from build123d import *
from OCP.BRepFilletAPI import BRepFilletAPI_MakeChamfer

# Parameters (mm, degrees)
BOSS_EXTRUDE1_DEPTH = 22
SKETCH2_R           = 7.95
BOSS_EXTRUDE2_DEPTH = 8
SKETCH3_OUTSIDE_W   = 32.288
SKETCH3_OUTSIDE_H   = 29.348
SKETCH3_OUTSIDE_R   = 9
CUT_EXTRUDE1_DEPTH  = 2
FILLET1_R           = 2
CHAMFER1_SIZE       = 2
FILLET2_R           = 2
CUT_EXTRUDE2_START  = -5
SKETCH4_OUTSIDE_W   = 31.604
SKETCH4_OUTSIDE_H   = 29.284
SKETCH4_OUTSIDE_R   = 8.5
CUT_EXTRUDE2_DEPTH  = 6
SKETCH5_R           = 4
CUT_EXTRUDE3_DEPTH  = 3
FILLET3_R           = 2
SKETCH6_R           = 5
CUT_EXTRUDE4_DEPTH  = 19
SKETCH7_R           = 0.7
CUT_EXTRUDE5_DEPTH  = 31.543264727
CHAMFER2_SIZE       = 0.5
CHAMFER2_SIZE2      = 0.288675135
SKETCH9_R           = 4
CUT_EXTRUDE6_DEPTH  = 31.543264727


with BuildPart() as part:
    # Sketch1 → Boss-Extrude1 (new body)
    with BuildSketch(Plane.XY):
        Polygon((10.969655115, 0), (5.484827557, 9.5), (-5.484827557, 9.5), (-10.969655115, 0), (-5.484827557, -9.5), (5.484827557, -9.5), align=None)
    extrude(amount=BOSS_EXTRUDE1_DEPTH)

    # Sketch2 → Boss-Extrude2 (add)
    with BuildSketch(Plane(origin=(0, 0, 0), x_dir=(-1, 0, 0), z_dir=(0, 0, -1))):
        Circle(SKETCH2_R)
    extrude(amount=BOSS_EXTRUDE2_DEPTH)

    # Sketch3 outside → Cut-Extrude1 (cut)
    with BuildSketch(Plane.XY.offset(22)):
        Rectangle(SKETCH3_OUTSIDE_W, SKETCH3_OUTSIDE_H)
        Circle(SKETCH3_OUTSIDE_R, mode=Mode.SUBTRACT)
    extrude(amount=-CUT_EXTRUDE1_DEPTH, mode=Mode.SUBTRACT)

    # Fillet1
    fillet1_edges = [part.edges().sort_by_distance(p)[0] for p in [
        (5.484827557, -9.5, 10),
        (-5.484827557, -9.5, 10),
        (-10.969655115, 0, 10),
        (-5.484827557, 9.5, 10),
        (5.484827557, 9.5, 10),
        (10.969655115, 0, 10),
    ]]
    fillet(fillet1_edges, radius=FILLET1_R)

    # Chamfer1
    # the kernel refuses this chamfer: 2 mm, written as the material it takes off along each edge
    with BuildSketch(Plane(origin=(-4.330127019, -9.5, 20), x_dir=(0, 1, 0), z_dir=(1, 0, 0))) as chamfer1_piece_1_section:
        Polygon((CHAMFER1_SIZE, 0), (0, -CHAMFER1_SIZE), (0, 0), align=None)
    chamfer1_piece_1 = extrude(amount=8.660254038, mode=Mode.PRIVATE)
    chamfer1_piece_1 = chamfer1_piece_1 - Plane(origin=(0, 0, 20), x_dir=(1, 0, 0), z_dir=(0, 0, 1)) * Cylinder(9, 26, mode=Mode.PRIVATE)
    add(chamfer1_piece_1, mode=Mode.SUBTRACT)
    with BuildSketch(Plane(origin=(4.330127019, -7.5, 20), x_dir=(0.8660254037844417, -0.49999999999999456, 0), z_dir=(0.49999999999999456, 0.8660254037844417, 0))) as chamfer1_piece_2_section:
        Polygon((2 - CHAMFER1_SIZE, 0), (2, CHAMFER1_SIZE), (2, 0), align=None)
    chamfer1_piece_2 = revolve(axis=Axis((4.330127019, -7.5, 20), (0, 0, -1)), revolution_arc=60, mode=Mode.PRIVATE)
    chamfer1_piece_2 = chamfer1_piece_2 - Plane(origin=(0, 0, 20), x_dir=(1, 0, 0), z_dir=(0, 0, 1)) * Cylinder(9, 8, mode=Mode.PRIVATE)
    add(chamfer1_piece_2, mode=Mode.SUBTRACT)
    with BuildSketch(Plane(origin=(-4.330127019, -7.5, 20), x_dir=(0, -1, 0), z_dir=(1, 0, 0))) as chamfer1_piece_3_section:
        Polygon((2 - CHAMFER1_SIZE, 0), (2, CHAMFER1_SIZE), (2, 0), align=None)
    chamfer1_piece_3 = revolve(axis=Axis((-4.330127019, -7.5, 20), (0, 0, -1)), revolution_arc=60, mode=Mode.PRIVATE)
    chamfer1_piece_3 = chamfer1_piece_3 - Plane(origin=(0, 0, 20), x_dir=(1, 0, 0), z_dir=(0, 0, 1)) * Cylinder(9, 8, mode=Mode.PRIVATE)
    add(chamfer1_piece_3, mode=Mode.SUBTRACT)
    with BuildSketch(Plane(origin=(6.062177826, -8.5, 20), x_dir=(-0.8660254037844416, 0.499999999999995, 0), z_dir=(0.499999999999995, 0.8660254037844416, 0))) as chamfer1_piece_4_section:
        Polygon((CHAMFER1_SIZE, 0), (0, -CHAMFER1_SIZE), (0, 0), align=None)
    chamfer1_piece_4 = extrude(amount=8.660254038, mode=Mode.PRIVATE)
    chamfer1_piece_4 = chamfer1_piece_4 - Plane(origin=(0, 0, 20), x_dir=(1, 0, 0), z_dir=(0, 0, 1)) * Cylinder(9, 26, mode=Mode.PRIVATE)
    add(chamfer1_piece_4, mode=Mode.SUBTRACT)
    with BuildSketch(Plane(origin=(-10.392304845, -1, 20), x_dir=(0.8660254037844345, 0.5000000000000072, 0), z_dir=(0.5000000000000072, -0.8660254037844346, 0))) as chamfer1_piece_5_section:
        Polygon((CHAMFER1_SIZE, 0), (0, -CHAMFER1_SIZE), (0, 0), align=None)
    chamfer1_piece_5 = extrude(amount=8.660254038, mode=Mode.PRIVATE)
    chamfer1_piece_5 = chamfer1_piece_5 - Plane(origin=(0, 0, 20), x_dir=(1, 0, 0), z_dir=(0, 0, 1)) * Cylinder(9, 26, mode=Mode.PRIVATE)
    add(chamfer1_piece_5, mode=Mode.SUBTRACT)
    with BuildSketch(Plane(origin=(8.660254038, 0, 20), x_dir=(0.866025403784438, 0.500000000000001, 0), z_dir=(-0.500000000000001, 0.866025403784438, 0))) as chamfer1_piece_6_section:
        Polygon((2, CHAMFER1_SIZE), (2 - CHAMFER1_SIZE, 0), (2, 0), align=None)
    chamfer1_piece_6 = revolve(axis=Axis((8.660254038, 0, 20), (0, 0, -1)), revolution_arc=60, mode=Mode.PRIVATE)
    chamfer1_piece_6 = chamfer1_piece_6 - Plane(origin=(0, 0, 20), x_dir=(1, 0, 0), z_dir=(0, 0, 1)) * Cylinder(9, 9, mode=Mode.PRIVATE)
    add(chamfer1_piece_6, mode=Mode.SUBTRACT)
    with BuildSketch(Plane(origin=(-8.660254038, 0, 20), x_dir=(-0.8660254037844414, 0.4999999999999952, 0), z_dir=(0.4999999999999952, 0.8660254037844414, 0))) as chamfer1_piece_7_section:
        Polygon((2 - CHAMFER1_SIZE, 0), (2, -CHAMFER1_SIZE), (2, 0), align=None)
    chamfer1_piece_7 = revolve(axis=Axis((-8.660254038, 0, 20), (0, 0, 1)), revolution_arc=60, mode=Mode.PRIVATE)
    chamfer1_piece_7 = chamfer1_piece_7 - Plane(origin=(0, 0, 20), x_dir=(1, 0, 0), z_dir=(0, 0, 1)) * Cylinder(9, 8, mode=Mode.PRIVATE)
    add(chamfer1_piece_7, mode=Mode.SUBTRACT)
    with BuildSketch(Plane(origin=(10.392304845, 1, 20), x_dir=(0, 0, -1), z_dir=(-0.500000000000001, 0.866025403784438, 0))) as chamfer1_piece_8_section:
        Polygon((CHAMFER1_SIZE, 0), (0, CHAMFER1_SIZE), (0, 0), align=None)
    chamfer1_piece_8 = extrude(amount=8.660254038, mode=Mode.PRIVATE)
    chamfer1_piece_8 = chamfer1_piece_8 - Plane(origin=(0, 0, 20), x_dir=(1, 0, 0), z_dir=(0, 0, 1)) * Cylinder(9, 26, mode=Mode.PRIVATE)
    add(chamfer1_piece_8, mode=Mode.SUBTRACT)
    with BuildSketch(Plane(origin=(-6.062177826, 8.5, 20), x_dir=(0.8660254037844415, -0.49999999999999517, 0), z_dir=(-0.49999999999999517, -0.8660254037844415, 0))) as chamfer1_piece_9_section:
        Polygon((CHAMFER1_SIZE, 0), (0, -CHAMFER1_SIZE), (0, 0), align=None)
    chamfer1_piece_9 = extrude(amount=8.660254038, mode=Mode.PRIVATE)
    chamfer1_piece_9 = chamfer1_piece_9 - Plane(origin=(0, 0, 20), x_dir=(1, 0, 0), z_dir=(0, 0, 1)) * Cylinder(9, 26, mode=Mode.PRIVATE)
    add(chamfer1_piece_9, mode=Mode.SUBTRACT)
    with BuildSketch(Plane(origin=(4.330127019, 7.5, 20), x_dir=(0.8660254037844379, 0.5000000000000013, 0), z_dir=(0.5000000000000013, -0.8660254037844379, 0))) as chamfer1_piece_10_section:
        Polygon((2, -CHAMFER1_SIZE), (2 - CHAMFER1_SIZE, 0), (2, 0), align=None)
    chamfer1_piece_10 = revolve(axis=Axis((4.330127019, 7.5, 20), (0, 0, 1)), revolution_arc=60, mode=Mode.PRIVATE)
    chamfer1_piece_10 = chamfer1_piece_10 - Plane(origin=(0, 0, 20), x_dir=(1, 0, 0), z_dir=(0, 0, 1)) * Cylinder(9, 9, mode=Mode.PRIVATE)
    add(chamfer1_piece_10, mode=Mode.SUBTRACT)
    with BuildSketch(Plane(origin=(-4.330127019, 7.5, 20), x_dir=(0, 1, 0), z_dir=(1, 0, 0))) as chamfer1_piece_11_section:
        Polygon((2 - CHAMFER1_SIZE, 0), (2, -CHAMFER1_SIZE), (2, 0), align=None)
    chamfer1_piece_11 = revolve(axis=Axis((-4.330127019, 7.5, 20), (0, 0, 1)), revolution_arc=60, mode=Mode.PRIVATE)
    chamfer1_piece_11 = chamfer1_piece_11 - Plane(origin=(0, 0, 20), x_dir=(1, 0, 0), z_dir=(0, 0, 1)) * Cylinder(9, 8, mode=Mode.PRIVATE)
    add(chamfer1_piece_11, mode=Mode.SUBTRACT)
    with BuildSketch(Plane(origin=(4.330127019, 9.5, 20), x_dir=(0, -1, 0), z_dir=(-1, 0, 0))) as chamfer1_piece_12_section:
        Polygon((CHAMFER1_SIZE, 0), (0, -CHAMFER1_SIZE), (0, 0), align=None)
    chamfer1_piece_12 = extrude(amount=8.660254038, mode=Mode.PRIVATE)
    chamfer1_piece_12 = chamfer1_piece_12 - Plane(origin=(0, 0, 20), x_dir=(1, 0, 0), z_dir=(0, 0, 1)) * Cylinder(9, 26, mode=Mode.PRIVATE)
    add(chamfer1_piece_12, mode=Mode.SUBTRACT)

    # Fillet2
    # the kernel refuses this fillet: 2 mm, written as the material it takes off along each edge
    with BuildSketch(Plane(origin=(0, 0, 22), x_dir=(1, 0, 0), z_dir=(0, -1, 0))) as fillet2_piece_1:
        with BuildLine():
            CenterArc((9 - FILLET2_R, -FILLET2_R), FILLET2_R, 0, 90)
            Line((9 - FILLET2_R, 0), (9, 0))
            Line((9, 0), (9, -FILLET2_R))
        make_face()
    revolve(axis=Axis((0, 0, 22), (0, 0, 1)), mode=Mode.SUBTRACT)

    # Sketch4 outside → Cut-Extrude2 (cut)
    with BuildSketch(Plane(origin=(0, 0, 0), x_dir=(-1, 0, 0), z_dir=(0, 0, -1)).offset(CUT_EXTRUDE2_START)):
        Rectangle(SKETCH4_OUTSIDE_W, SKETCH4_OUTSIDE_H)
        Circle(SKETCH4_OUTSIDE_R, mode=Mode.SUBTRACT)
    extrude(amount=-CUT_EXTRUDE2_DEPTH, mode=Mode.SUBTRACT)

    # Sketch5 → Cut-Extrude3 (cut)
    with BuildSketch(Plane.XY.offset(22)):
        Circle(SKETCH5_R)
    extrude(amount=-CUT_EXTRUDE3_DEPTH, mode=Mode.SUBTRACT)

    # Fillet3
    fillet3_edges = [part.edges().sort_by_distance(p)[0] for p in [
        (-4, 0, 22),
    ]]
    fillet(fillet3_edges, radius=FILLET3_R)

    # Sketch6 → Cut-Extrude4 (cut)
    with BuildSketch(Plane(origin=(0, 0, -8), x_dir=(-1, 0, 0), z_dir=(0, 0, -1))):
        Circle(SKETCH6_R)
    extrude(amount=-CUT_EXTRUDE4_DEPTH, mode=Mode.SUBTRACT)

    # Sketch7 → Cut-Extrude5 (cut, through all)
    with BuildSketch(Plane.XY.offset(19)):
        with Locations((-2.5, 0)):
            Circle(SKETCH7_R)
        with Locations((-1.25, 2.165063509)):
            Circle(SKETCH7_R)
        with Locations((1.25, 2.165063509)):
            Circle(SKETCH7_R)
        with Locations((2.5, 0)):
            Circle(SKETCH7_R)
        with Locations((1.25, -2.165063509)):
            Circle(SKETCH7_R)
        with Locations((-1.25, -2.165063509)):
            Circle(SKETCH7_R)
    extrude(amount=-CUT_EXTRUDE5_DEPTH, mode=Mode.SUBTRACT)

    # Sketch8 → Cut-Revolve1 (revolve, cut)
    with BuildSketch(Plane(origin=(0, 0, 0), x_dir=(1, 0, 0), z_dir=(0, 1, 0)), mode=Mode.PRIVATE) as cut_revolve1_sk:
        with BuildLine():
            Line((-6.75, 0.875), (-7.95, 0.875))
            Line((-7.95, 0.875), (-7.95, -0.625))
            Line((-7.95, -0.625), (-6.75, -0.625))
            ThreePointArc((-6.75, -0.625), (-6, 0.125), (-6.75, 0.875))
        make_face()
    revolve(cut_revolve1_sk.sketch.rotate(Axis((0, 0, 0), (0, 0, -1)), 180), axis=Axis((0, 0, 0), (0, 0, -1)), mode=Mode.SUBTRACT)

    # Chamfer2: one chamfer whose edges measure the first distance from different faces: ONE call of the kernel's chamfer builder (chamfer() names one face for all edges)
    chamfer2_edges_1 = [part.edges().sort_by_distance(p)[0] for p in [
        (-7.95, 0, 0),
    ]]
    chamfer2_side_1 = [part.faces().sort_by_distance(p)[0] for p in [
        (7.979921088, 4.607209589, 0),
    ]]
    chamfer2_edges_2 = [part.edges().sort_by_distance(p)[0] for p in [
        (7.95, 0, -0.875),
    ]]
    chamfer2_side_2 = [part.faces().sort_by_distance(p)[0] for p in [
        (7.95, 0, -4.4375),
    ]]
    chamfer2 = BRepFilletAPI_MakeChamfer(part.part.solid().wrapped)
    for e in chamfer2_edges_1:
        chamfer2.Add(CHAMFER2_SIZE, CHAMFER2_SIZE2, e.wrapped, chamfer2_side_1[0].wrapped)  # the first distance lies on this face
    for e in chamfer2_edges_2:
        chamfer2.Add(CHAMFER2_SIZE, CHAMFER2_SIZE2, e.wrapped, chamfer2_side_2[0].wrapped)  # the first distance lies on this face
    add(Compound.cast(chamfer2.Shape()), mode=Mode.REPLACE)

    # Sketch9 → Cut-Extrude6 (cut, through all)
    with BuildSketch(Plane.XY.offset(19)):
        Circle(SKETCH9_R)
    extrude(amount=-CUT_EXTRUDE6_DEPTH, mode=Mode.SUBTRACT)


solid = part.part
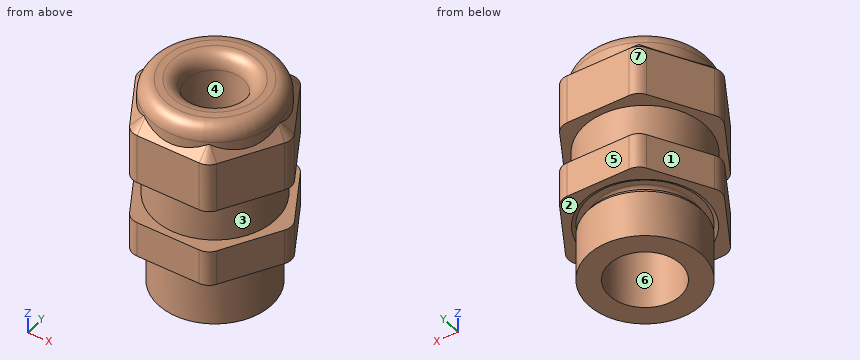
Here's how the part is built. I have some questions about the finished solid (model axes, mm). Face numbers are marked on the shaded views. A direction names the side the tool comes from. Coordinates: 2 decimals unless noted, no trailing zeros. Write each loop counter-clockwise with the first axis right and the second up, starting at its lowest first coordinate (ties: lowest second). Pieces come first, ordered by that corner, then holes. Notation, with made-up numbers: (7, 19) - (63, 19) arc R32 cw to (63, 58) - close; hole circle Ø10 at (24, -26.75). An arc over 180 degrees is marked (long way). Use one line per item in the form item = value.
1) I'm going to push flat-ended pins straight in: P1, Ø10.5, axis at x = 0, y = 0, coming from the +Z side; P2, Ø10, axis at y = 6.5, z = 15, coming from the +X side; P3, Ø2, axis at y = -2, z = 5, coming from the +X side. Where does each tip first touch, or does it pass through?
Solved:
P1 = 21.85
P2 = 10.1
P3 = 10.39
2) I need wall thicknesses on line 1 (Y direction, x = 0, z = 0.4); line 2 (Y direction, x = 0, z = 17.5); line 3 (Y direction, x = 0, z = 6.25). Which ranges of each line are inside material? Lowest first, please.
Solved:
line_1 = -9.5 to -7.95, -6.21 to -5, 5 to 6.21, 7.95 to 9.5
line_2 = -9.5 to -4, 4 to 9.5
line_3 = -8.5 to -5, 5 to 8.5
3) Suppose I cut it at A-A, the plane z = 2. Write out the boundary of the cut face in (x, y), plus the area to 3 significant figures.
Solved:
outline = (-10.39, -1) - (-6.06, -8.5) arc R2 ccw to (-4.33, -9.5) - (4.33, -9.5) arc R2 ccw to (6.06, -8.5) - (10.39, -1) arc R2 ccw to (10.39, 1) - (6.06, 8.5) arc R2 ccw to (4.33, 9.5) - (-4.33, 9.5) arc R2 ccw to (-6.06, 8.5) - (-10.39, 1) arc R2 ccw to start; hole circle Ø10 at (0, 0)
area = 233 mm2
4) Thinking about a two-plate mould opening in X: for the marked faces 4, 5, 6 and 7, which applies, released by +X, released by -X, zero draft, split by the parting line, or undercut?
Solved:
face_4 = undercut
face_5 = zero draft
face_6 = undercut
face_7 = released by -X
5) On a 3-axis mill with a long thin cutter (end or side, diameter ignored), from which of +Z, -Z, +X, -X, +Y, -Y can I reach the whole of each face in a straight line? I mean the marked faces 1, 2 and 3. Say none if no direction works.
Solved:
face_1 = +Z, -Z, -X, +Y
face_2 = -Z
face_3 = none
